Read the model definition and answer for the solid it produces. Units are mm, in the model's axes. Face numbers are marked on the shaded views. A direction names the side the tool comes from. Round coordinates to 2 decimals unless told otherwise and drop trailing zeros. Write each loop counter-clockwise with the first axis right and the second up, starting at its lowest first coordinate (ties: lowest second). Pieces come first, ordered by that corner, then holes. Notation, with made-up numbers: (72, 81) -> (103, 81) arc R24 cw to (103, 102) -> close; hole circle Ø4 at (28, 58). An arc over 180 degrees is marked (long way). Return JSON: item names as keys, results as strings.
from build123d import *

# Parameters (mm, degrees)
CROQUIS1_W                       = 1396
CROQUIS1_H                       = 392.64
BRIDA_BASE1_DEPTH                = 3.175
TALADRO_DE_MARGEN_PARA_1_41_D    = 6.7564
BRIDA_DE_ARISTA1_STRIP_W         = 32.7
BRIDA_DE_ARISTA1_STRIP_H         = 3.175
BRIDA_DE_ARISTA1_STRIP_CUT_DEPTH = 1396
BRIDA_DE_ARISTA1_DEPTH           = 1396
TALADRO_DE_MARGEN_PARA_1_42_D    = 6.7564
CROQUIS9_W                       = 1396
CROQUIS9_H                       = 20
CORTAR_EXTRUIR1_DEPTH            = 10


# Sheet-metal steps are written as plain solids
with BuildPart() as part:
    # Croquis1 → Brida base1 (new body)
    with BuildSketch(Plane(origin=(0, 0, 0), x_dir=(1, 0, 0), z_dir=(0, 1, 0))):
        with Locations((-11.780590717, 232.198987342)):
            Rectangle(CROQUIS1_W, CROQUIS1_H)
    extrude(amount=-BRIDA_BASE1_DEPTH)

    # Taladro de margen para 1/41 (through all)
    with Locations(Plane(origin=(0, -3.175, 0), x_dir=(-1, 0, 0), z_dir=(0, -1, 0))):
        with Locations((511.780590717, 161.278987342), (511.780590717, 335.878987342), (311.780590717, 161.278987342), (311.780590717, 335.878987342), (111.780590717, 161.278987342), (111.780590717, 335.878987342), (-88.219409283, 161.278987342), (-88.219409283, 335.878987342), (-288.219409283, 161.278987342), (-288.219409283, 335.878987342), (-488.219409283, 161.278987342), (-488.219409283, 335.878987342), (670.780590717, 161.278987342), (670.780590717, 335.878987342), (-647.219409283, 161.278987342), (-647.219409283, 335.878987342)):
            Hole(TALADRO_DE_MARGEN_PARA_1_41_D / 2)

    # Brida de arista1 strip (across the edge) → Brida de arista1 strip cut (cut)
    with BuildSketch(Plane(origin=(-709.780590717, -3.175, -428.518987342), x_dir=(0, 0, 1), z_dir=(1, 0, 0))):
        with Locations((-3.175, -1.5875)):
            Rectangle(BRIDA_DE_ARISTA1_STRIP_W, BRIDA_DE_ARISTA1_STRIP_H)
    extrude(amount=BRIDA_DE_ARISTA1_STRIP_CUT_DEPTH, mode=Mode.SUBTRACT)

    # Brida de arista1 section (across the edge) → Brida de arista1 (add)
    with BuildSketch(Plane(origin=(-709.780590717, -3.175, -428.518987342), x_dir=(0, 0, 1), z_dir=(1, 0, 0))):
        with BuildLine():
            Line((0, 10), (0, 56.825))
            Line((0, 56.825), (3.175, 56.825))
            Line((3.175, 56.825), (3.175, 10))
            ThreePointArc((3.175, 10), (6.103932188, 2.928932188), (13.175, 0))
            Line((13.175, 0), (13.175, -3.175))
            ThreePointArc((13.175, -3.175), (3.858868158, 0.683868158), (0, 10))
        make_face()
    extrude(amount=BRIDA_DE_ARISTA1_DEPTH)

    # Taladro de margen para 1/42 (through all)
    with Locations(Plane.XY.offset(-425.343987342)):
        with Locations((-425.550590717, -32.4), (-260.180590717, -32.4), (-94.810590717, -32.4), (70.559409283, -32.4), (235.929409283, -32.4), (401.299409283, -32.4)):
            Hole(TALADRO_DE_MARGEN_PARA_1_42_D / 2)

    # Croquis9 → Cortar-Extruir1 (cut)
    with BuildSketch(Plane(origin=(0, -3.175, 0), x_dir=(-1, 0, 0), z_dir=(0, -1, 0))):
        with Locations((11.780590717, 45.878987342)):
            Rectangle(CROQUIS9_W, CROQUIS9_H)
    extrude(amount=-CORTAR_EXTRUIR1_DEPTH, mode=Mode.SUBTRACT)


solid = part.part
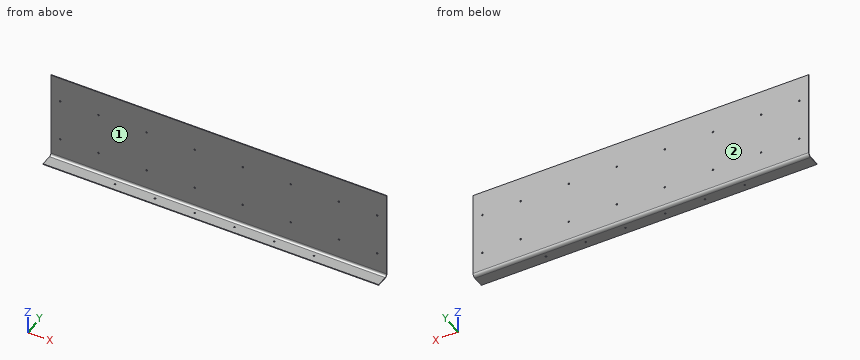
Item 1: Section C-C (y = -48) is taken. Give the vertices of the cut face in (x, z), then the cut area to 3 significant figures.
Worked answers:
{"outline": "(-709.78, -428.52) -> (686.22, -428.52) -> (686.22, -425.34) -> (-709.78, -425.34) -> close", "area": "4,430 mm2"}
Item 2: Straight lines are drawn through the part: L1, parallel to Y at x = -114, z = -263.5 (3 decimals); L2, parallel to Z at x = 36, y = -12.5; L3, parallel to Z at x = 395, y = -11.5. For each, find the intervals that lie inside material, in ascending order. Write a range as [from, to].
Worked answers:
{"L1": "y = [-3.175, 0]", "L2": "z = [-428.5, -425.32]", "L3": "z = [-428.41, -425.2]"}
Item 3: Section B-B (z = -200) is taken. Give the vertices of the cut face in (x, y) (3 decimals), then the cut area to 3 significant figures.
Worked answers:
{"outline": "(-709.781, -3.175) -> (686.219, -3.175) -> (686.219, 0) -> (-709.781, 0) -> close", "area": "4,430 mm2"}
Item 4: Section A-A (x = 583.5) is taken. Give the vertices of the cut face in (y, z) (3 decimals).
Worked answers:
{"outline": "(-60, -428.519) -> (-13.175, -428.519) arc R13.175 ccw to (0, -415.344) -> (0, -55.879) -> (-3.175, -55.879) -> (-3.175, -415.344) arc R10 cw to (-13.175, -425.344) -> (-60, -425.344) -> close"}
Item 5: Flat-ended cylindrical pins translate along their axes: pin 1 (2 mm diameter, centred on x = 88.5, z = -367, fed in from -Y) (3 decimals); pin 2 (8 mm diameter, centred on x = 488.22, z = -335.88, fed in from +Y); pin 3 (6 mm diameter, centred on x = -378, y = -14, fed in from +Z); pin 4 (4 mm diameter, centred on x = -193, y = -24, fed in from +Z). Find the tip coordinate at first contact, or state that the pin passes through.
Worked answers:
{"pin 1": "stops at y = -3.175", "pin 2": "stops at y = 0", "pin 3": "stops at z = -425.1", "pin 4": "stops at z = -425.34"}
Item 6: A tool of negligible diameter and unlimited length cuts with its end or side. For the marked faces 1 and 2, from which of +Z, -Z, +X, -X, +Y, -Y can it reach the whole face along a straight path? Write none if from no direction.
Worked answers:
{"face 1": "+Z, +X, -X, -Y", "face 2": "+Z, -Z, +X, -X, +Y"}
